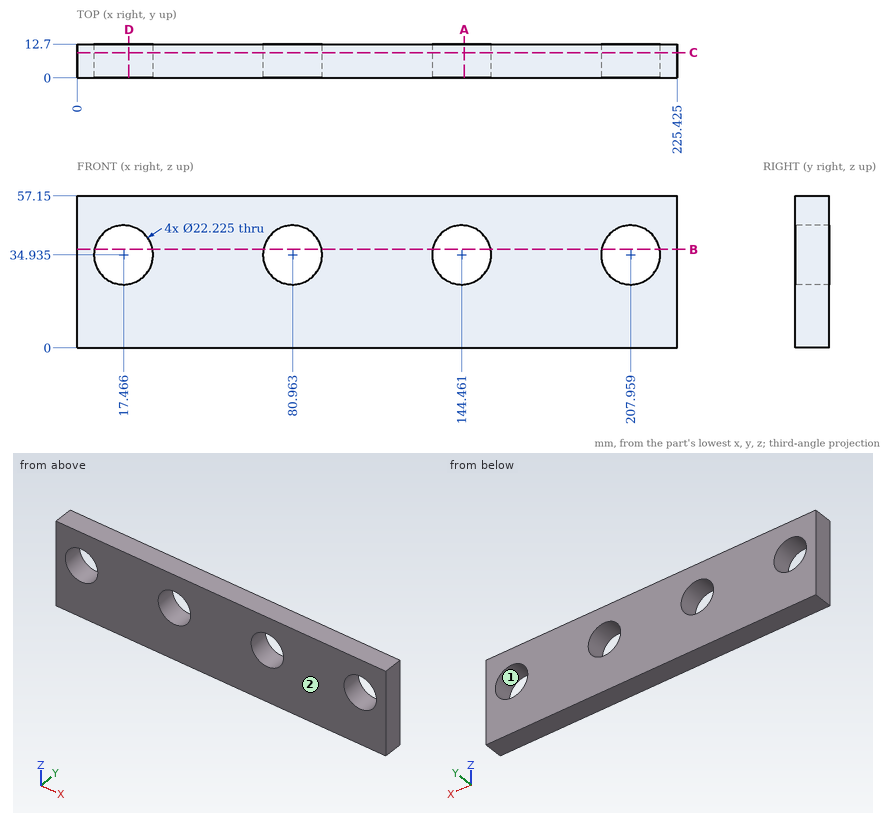
Study the drawing (mm; zero at the part's minimum x, y, z) and answer. Coordinates: 2 decimals unless noted, no trailing zeros. Write each loop counter-clockwise with the first axis right and the second up, starting at its lowest first coordinate (ties: lowest second). Pieces come first, ordered by that corner, then holes.
Q1. A cutting plane is placed at D-D, the plane x = 19.5. Give the vertices of the cut face in (y, z).
Q2. A cutting plane is placed at C-C, the plane y = 9.5. State how many separate pieces and enclosed holes the cut face has, then the cut area to 3 significant figures.
Q3. Find the intervals of material crossed by line 1 (X direction, y = 0.75, z = 34) (1 decimal); line 2 (X direction, y = 5.25, z = 38) (1 decimal), in increasing order.
Q4. Determine the mould class of the marked faces 1 and 2 for opening direction Z: released by +Z, released by -Z, zero draft, split by the parting line, or undercut.
Q5. A cutting plane is placed at A-A, the plane x = 145.5. Give the vertices of the cut face in (y, z), then the cut area to 3 significant figures.
Q6. A cutting plane is placed at B-B, the plane z = 37. Give the vertices of the cut face in (x, y) (1 decimal).
Findings below:
1. outline: (0, 0) - (12.7, 0) - (12.7, 24.01) - (0, 24.01) - close; (0, 45.86) - (12.7, 45.86) - (12.7, 57.15) - (0, 57.15) - close
2. separate pieces: 1
2. enclosed holes: 4
2. area: 11,300 mm2
3. line 1: x = 0 to 6.4, 28.5 to 69.9, 92 to 133.4, 155.5 to 196.9, 219 to 225.4
3. line 2: x = 0 to 6.8, 28.1 to 70.3, 91.6 to 133.8, 155.1 to 197.3, 218.6 to 225.4
4. face 1: undercut
4. face 2: zero draft
5. outline: (0, 0) - (12.7, 0) - (12.7, 23.87) - (0, 23.87) - close; (0, 46) - (12.7, 46) - (12.7, 57.15) - (0, 57.15) - close
5. area: 445 mm2
6. outline: (0, 0) - (6.5, 0) - (6.5, 12.7) - (0, 12.7) - close; (28.4, 0) - (70, 0) - (70, 12.7) - (28.4, 12.7) - close; (91.9, 0) - (133.5, 0) - (133.5, 12.7) - (91.9, 12.7) - close; (155.4, 0) - (197, 0) - (197, 12.7) - (155.4, 12.7) - close; (218.9, 0) - (225.4, 0) - (225.4, 12.7) - (218.9, 12.7) - close
